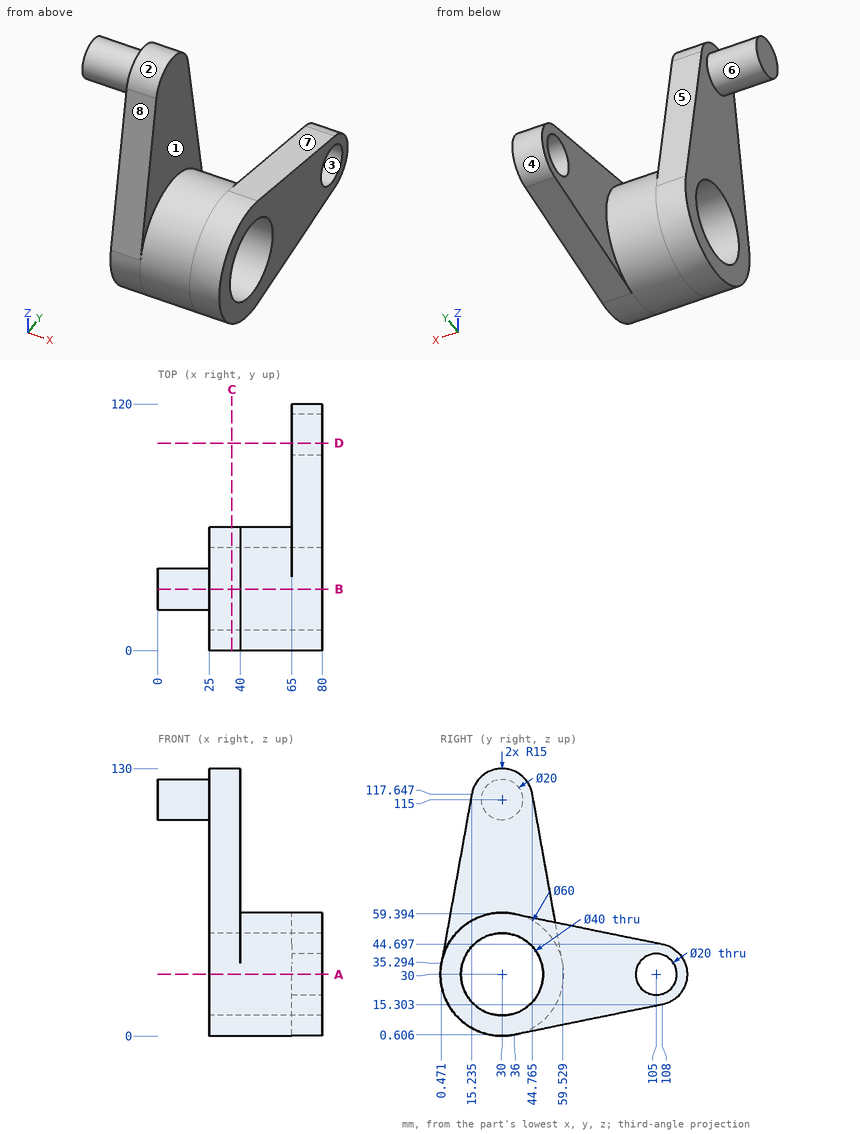
The figure shows three views and two pictorial views of one solid part (mm, origin at its lowest corner). Answer the questions. A direction names the side the tool comes from. Coordinates: 2 decimals unless noted, no trailing zeros. Loops run counter-clockwise (first coordinate to the right, second up) from the corner with the lowest first, then second, coordinate; pieces in that order, holes last.
(1) Flat-ended cylindrical pins translate along their axes: pin 1 Ø10 at (y, z) = (38.5, 93) entering from +X; pin 2 Ø16 at (y, z) = (105, 30) entering from +X; pin 3 Ø10 at (x, y) = (38.5, 19) entering from -Z; pin 4 Ø17.5 at (y, z) = (71.5, 40.5) entering from -X. Find the tip coordinate at first contact, or state that the pin passes through.
Solution:
pin 1: stops at x = 40
pin 2: passes through
pin 3: stops at z = 0.61
pin 4: stops at x = 65
(2) Consider line 1 along Y through (x, z) = (70.5, 30); line 2 along Y through (x, z) = (39, 30). Determine where each line is inside the solid, lowest interval first.
Solution:
line 1: y = 0 to 10, 50 to 95, 115 to 120
line 2: y = 0 to 10, 50 to 60
(3) The part is cut by section B-B (y = 30). Determine the outline of the cut face in (x, z), and give its area (3 significant figures).
Solution:
outline: (0, 105) - (25, 105) - (25, 50) - (80, 50) - (80, 60) - (40, 60) - (40, 130) - (25, 130) - (25, 125) - (0, 125) - close; (25, 0) - (80, 0) - (80, 10) - (25, 10) - close
area: 2,650 mm2
(4) The part is cut by section D-D (y = 101). Determine the outline of the cut face in (x, z) (1 decimal), and give its area (3 significant figures).
Solution:
outline: (65, 13.9) - (80, 13.9) - (80, 20.8) - (65, 20.8) - close; (65, 39.2) - (80, 39.2) - (80, 46.1) - (65, 46.1) - close
area: 209 mm2
(5) The mould has two halves that part along Z. Classify the marked faces 1, 2, 3 and 4: released by +Z, released by -Z, zero draft, split by the parting line, or undercut.
Solution:
face 1: zero draft
face 2: released by +Z
face 3: undercut
face 4: split by the parting line
(6) A tool of negligible diameter and unlimited length cuts with its end or side. For the marked faces 5, 6, 7 and 8, from which of +Z, -Z, +X, -X, +Y, -Y can it reach the whole face along a straight path? Write none if from no direction.
Solution:
face 5: +Z, -X, +Y
face 6: -X
face 7: +Z, +X, +Y
face 8: +Z, +X, -X, -Y
(7) The part is cut by section C-C (x = 36). Determine the outline of the cut face in (y, z) (1 decimal).
Solution:
outline: (0.5, 35.3) arc R30 ccw (long way) to (59.5, 35.3) - (44.8, 117.6) arc R15 ccw to (15.2, 117.6) - close; hole circle Ø40 at (30, 30)
(8) The part is cut by section A-A (z = 30). Determine the outline of the cut face in (x, y), and give its area (3 significant figures).
Solution:
outline: (25, 0) - (80, 0) - (80, 10) - (25, 10) - close; (25, 50) - (80, 50) - (80, 95) - (65, 95) - (65, 60) - (25, 60) - close; (65, 115) - (80, 115) - (80, 120) - (65, 120) - close
area: 1,700 mm2
